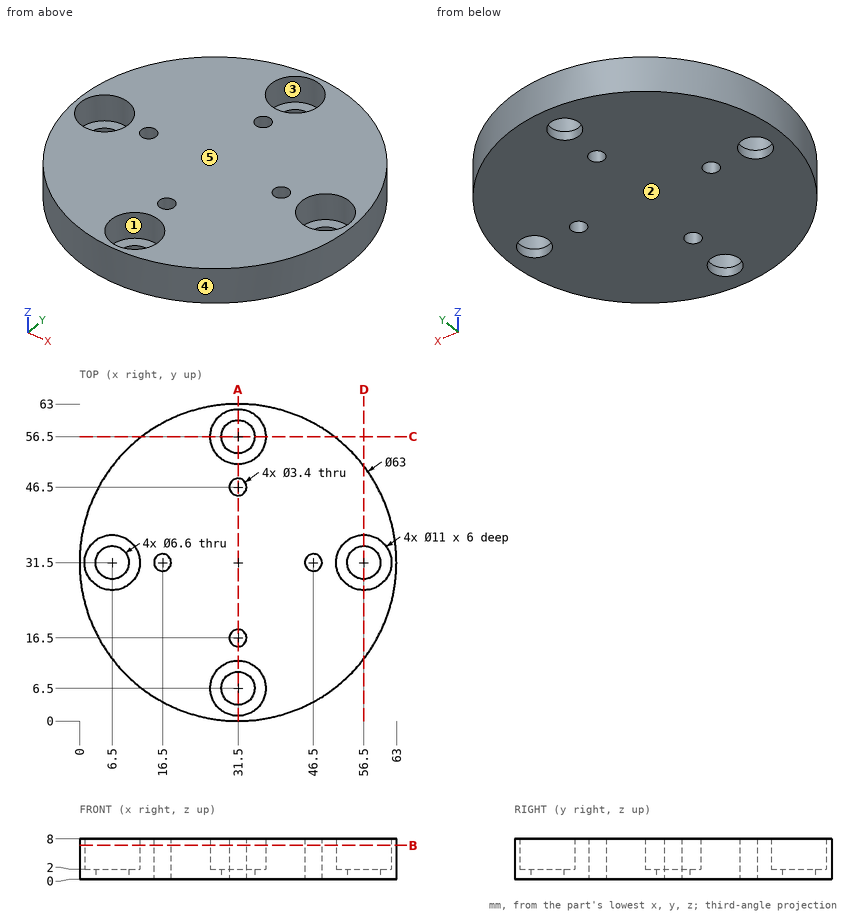
Design review of the part shown in the three views and the two pictorial views. Dimensions are in mm from the part's minimum x, y and z. A direction names the side the tool comes from. Coordinates: 2 decimals unless noted, no trailing zeros. Write each loop counter-clockwise with the first axis right and the second up, starting at its lowest first coordinate (ties: lowest second). Pieces come first, ordered by that corner, then holes.
1) Clearance check with flat-ended pins moving along their axes: pin 1 Ø5.5 at (x, y) = (31.5, 56.5) entering from +Z; pin 2 Ø1.5 at (y, z) = (43.5, 2) entering from -X; pin 3 Ø4 at (y, z) = (46.5, 7) entering from +X; pin 4 Ø1 at (y, z) = (52.5, 4.5) entering from -X. State where each tip first meets the part, or that it passes through.
2) We need section C-C on y = 56.5. State the section outline as (x, z) points.
3) We need section A-A on x = 31.5. State the section outline as (y, z) points.
4) Machinability: for the marked faces 1 and 2, which of the approach directions +Z, -Z, +X, -X, +Y, -Y give a long, thin tool a straight path to every point of the face, cutting with its end or side? Answer none if there is none.
5) We need section B-B on z = 6.75. Count the separate pieces of the cut face and the enclosed holes in it, then the cut area to 3 significant figures.
6) The part is to be moulded in two halves that separate along X. For the marked faces 3, 4 and 5, say which applies: pulls with the +X half, pulls with the -X half, needs draft (parallel to the pull), parting line crosses it, or undercut.
7) To check wall thickness, follow probe 1 along Y at (x, z) = (31.5, 1.25); probe 2 along Y at (x, z) = (27.5, 4) (3 decimals); probe 3 along X at (y, z) = (35, 3.25). State the ranges of each line that lie inside material, in increasing order.
Answer list:
1. pin 1: passes through
1. pin 2: stops at x = 2.08
1. pin 3: stops at x = 60.19
1. pin 4: stops at x = 7.58
2. outline: (12.34, 0) - (28.2, 0) - (28.2, 2) - (26, 2) - (26, 8) - (12.34, 8) - close; (34.8, 0) - (50.66, 0) - (50.66, 8) - (37, 8) - (37, 2) - (34.8, 2) - close
3. outline: (0, 0) - (3.2, 0) - (3.2, 2) - (1, 2) - (1, 8) - (0, 8) - close; (9.8, 0) - (14.8, 0) - (14.8, 8) - (12, 8) - (12, 2) - (9.8, 2) - close; (18.2, 0) - (44.8, 0) - (44.8, 8) - (18.2, 8) - close; (48.2, 0) - (53.2, 0) - (53.2, 2) - (51, 2) - (51, 8) - (48.2, 8) - close; (59.8, 0) - (63, 0) - (63, 8) - (62, 8) - (62, 2) - (59.8, 2) - close
4. face 1: +Z
4. face 2: -Z, +X, -X, +Y, -Y
5. separate pieces: 1
5. enclosed holes: 8
5. area: 2,700 mm2
6. face 3: undercut
6. face 4: parting line crosses it
6. face 5: needs draft
7. probe 1: y = 0 to 3.2, 9.8 to 14.8, 18.2 to 44.8, 48.2 to 53.2, 59.8 to 63
7. probe 2: y = 0.255 to 2.725, 10.275 to 52.725, 60.275 to 62.745
7. probe 3: x = 0.2 to 2.26, 10.74 to 52.26, 60.74 to 62.8
